The drawing under review shows one solid part. Ordinate dimensions are in mm from its lowest x, y, z. Coordinates: 2 decimals unless noted, no trailing zeros. Order: outer loops, then holes, each group sorted by start corner. A loop starts at its lowest first (then second) coordinate and runs counter-clockwise, first axis right, second up.
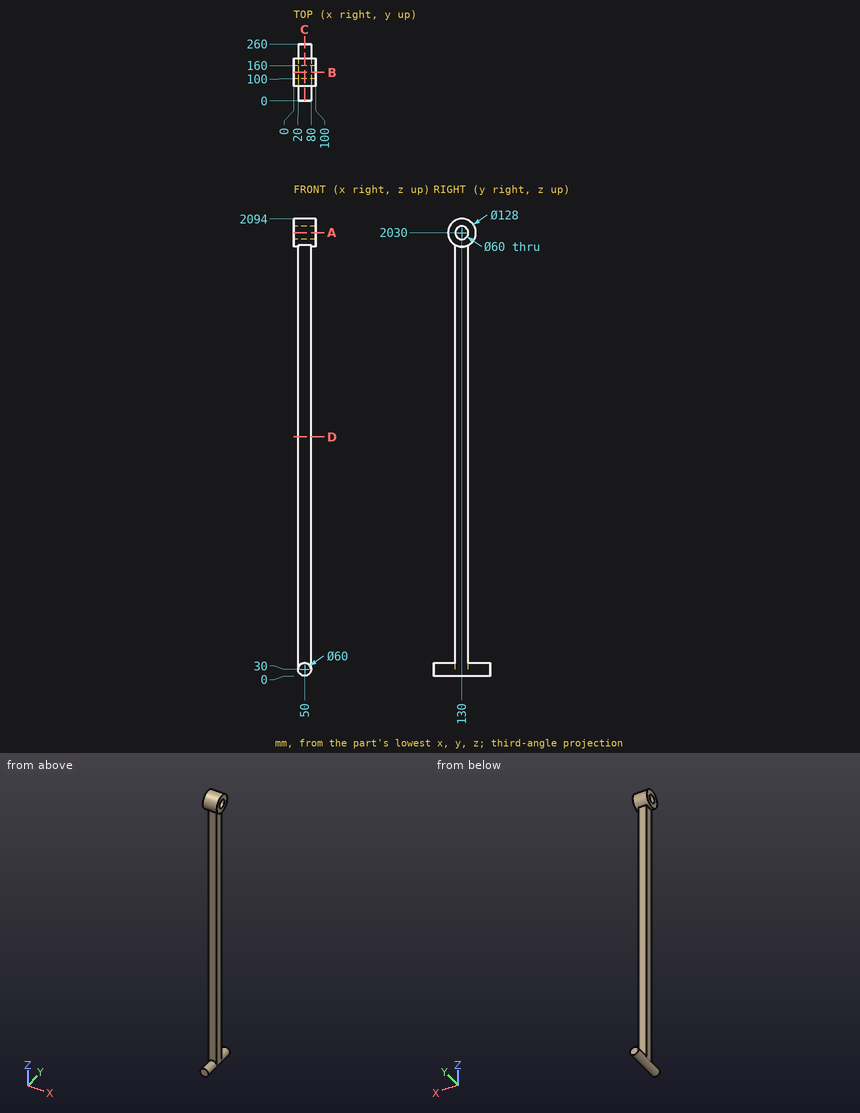
1. Take a section at D-D, the plane z = 1095.5. Give the boundary of the cut face in (x, y), plus the area to 3 significant figures.
Answer below:
outline: (20, 100) - (80, 100) - (80, 160) - (20, 160) - close
area: 3,600 mm2
2. Clearance check with flat-ended pins moving along their axes: pin 1 Ø3 at (x, y) = (18.5, 95) entering from +Z; pin 2 Ø2 at (x, z) = (37.5, 558) entering from -Y; pin 3 Ø12 at (x, z) = (85.5, 967) entering from +Y. State where each tip first meets the part, or that it passes through.
Answer below:
pin 1: stops at z = 2084.53
pin 2: stops at y = 100
pin 3: stops at y = 160
3. To check wall thickness, follow L1, parallel to Z at x = 55, y = 129; L2, parallel to X at y = 115.5, z = 1323.5; L3, parallel to Z at x = 56.5, y = 115. State the ranges of each line that lie inside material, in increasing order.
Answer below:
L1: z = 0.42 to 2000.02, 2059.98 to 2093.99
L2: x = 20 to 80
L3: z = 0.71 to 2004.02, 2055.98 to 2092.22
4. Take a section at C-C, the plane x = 50. Give the boundary of the cut face in (y, z), plus the area to 3 significant figures.
Answer below:
outline: (0, 0) - (260, 0) - (260, 60) - (160, 60) - (160, 1973.47) arc R64 ccw (long way) to (100, 1973.47) - (100, 60) - (0, 60) - close; hole circle Ø60 at (130, 2030)
area: 140,000 mm2
5. Take a section at B-B, the plane y = 130. Give the boundary of the cut face in (x, z).
Answer below:
outline: (0, 1966) - (20, 1966) - (20, 30) arc R30 ccw to (80, 30) - (80, 1966) - (100, 1966) - (100, 2000) - (0, 2000) - close; (0, 2060) - (100, 2060) - (100, 2094) - (0, 2094) - close
6. Take a section at A-A, the plane z = 2030. Give the boundary of the cut face in (x, y).
Answer below:
outline: (0, 66) - (100, 66) - (100, 100) - (0, 100) - close; (0, 160) - (100, 160) - (100, 194) - (0, 194) - close
